For this review, take the finished solid that the model builds, in its own axes (mm). A direction names the side the tool comes from. Give positions to 0.01 mm unless a question says otherwise; leave off trailing zeros. Order: outer loops, then holes, each group sorted by start corner. A loop starts at its lowest first (then second) coordinate and runs counter-clockwise, first axis right, second up.
from build123d import *

# Parameters (mm, degrees)
SKETCH2_R               = 1.778
BOSS_EXTRUDE1_DEPTH     = 22.352
CUT_EXTRUDE1_DEPTH      = 186.610228447
CUT_EXTRUDE1_DEPTH_BACK = 186.610228447
SKETCH3_W               = 63.5
SKETCH3_H               = 9.652


with BuildPart() as part:
    # Sketch2 → Boss-Extrude1 (new body)
    with BuildSketch(Plane.XY):
        with BuildLine():
            Line((0, 6.35), (177.8, 6.35))
            ThreePointArc((177.8, 6.35), (184.15, 0), (177.8, -6.35))
            Line((177.8, -6.35), (0, -6.35))
            ThreePointArc((0, -6.35), (-6.35, 0), (0, 6.35))
        make_face()
        Circle(SKETCH2_R, mode=Mode.SUBTRACT)
        with Locations((25.4, 0)):
            Circle(SKETCH2_R, mode=Mode.SUBTRACT)
        with Locations((38.1, 0)):
            Circle(SKETCH2_R, mode=Mode.SUBTRACT)
        with Locations((50.8, 0)):
            Circle(SKETCH2_R, mode=Mode.SUBTRACT)
        with Locations(Location((127, 0, 0), (0, 0, 180))):
            Circle(SKETCH2_R, mode=Mode.SUBTRACT)
        with Locations(Location((139.7, 0, 0), (0, 0, 180))):
            Circle(SKETCH2_R, mode=Mode.SUBTRACT)
        with Locations(Location((152.4, 0, 0), (0, 0, 180))):
            Circle(SKETCH2_R, mode=Mode.SUBTRACT)
        with Locations(Location((177.8, 0, 0), (0, 0, 180))):
            Circle(SKETCH2_R, mode=Mode.SUBTRACT)
    extrude(amount=BOSS_EXTRUDE1_DEPTH)

    # Sketch3 → Cut-Extrude1 (cut, two sides: drawn at the far end of the back side and taken through both)
    with BuildSketch(Plane(origin=(0, 0, 0), x_dir=(1, 0, 0), z_dir=(0, 1, 0)).offset(-CUT_EXTRUDE1_DEPTH_BACK)):
        with Locations((25.4, -11.176)):
            Rectangle(SKETCH3_W, SKETCH3_H)
        with Locations((152.4, -11.176)):
            Rectangle(SKETCH3_W, SKETCH3_H)
    extrude(amount=CUT_EXTRUDE1_DEPTH + CUT_EXTRUDE1_DEPTH_BACK, mode=Mode.SUBTRACT)


solid = part.part
1) Clearance check with flat-ended pins moving along their axes: pin 1 (3 mm diameter, centred on y = 3, z = 13.5, fed in from +X); pin 2 (2 mm diameter, centred on x = 177.8, y = 0, fed in from +Z); pin 3 (1 mm diameter, centred on y = -0.5, z = 15, fed in from -X); pin 4 (2 mm diameter, centred on y = -4, z = 17, fed in from +X). State where each tip first meets the part, or that it passes through.
Answer sheet:
pin 1: stops at x = 120.65
pin 2: passes through
pin 3: stops at x = 57.15
pin 4: stops at x = 183.4
2) We need section B-B on x = 152.4. Give the boundary of the cut face in (y, z).
Answer sheet:
outline: (-6.35, 0) - (-1.78, 0) - (-1.78, 6.35) - (-6.35, 6.35) - close; (-6.35, 16) - (-1.78, 16) - (-1.78, 22.35) - (-6.35, 22.35) - close; (1.78, 0) - (6.35, 0) - (6.35, 6.35) - (1.78, 6.35) - close; (1.78, 16) - (6.35, 16) - (6.35, 22.35) - (1.78, 22.35) - close
3) We need section A-A on x = 11. Give the boundary of the cut face in (y, z).
Answer sheet:
outline: (-6.35, 0) - (6.35, 0) - (6.35, 6.35) - (-6.35, 6.35) - close; (-6.35, 16) - (6.35, 16) - (6.35, 22.35) - (-6.35, 22.35) - close
4) Draft analysis for pull direction X (two halves, no side actions). For faces 1 (the face through (184.15, 0.14, 19.13)), 2 (the face through (57.15, 0, 11)), 3 (the face through (154.176, -0.078, 19.133)), 4 (the face through (25, -3, 16.002)), state which applies: +X half, -X half, draft (parallel to the pull), parting line (faces both ways), or undercut.
Answer sheet:
face 1: +X half
face 2: -X half
face 3: undercut
face 4: draft
5) Tool access review of faces 5 (the face through (152, -3, 16.002)), 6 (the face through (90, 0, 0)): name each direction out of +Z, -Z, +X, -X, +Y, -Y from which nothing blocks a thin tool from reaching the whole face with its end or side.
Answer sheet:
face 5: +X, +Y, -Y
face 6: -Z, +X, -X, +Y, -Y
6) We need section C-C on y = 0. Count the separate pieces of the cut face and the enclosed holes in it, then the cut area to 3 significant figures.
Answer sheet:
separate pieces: 17
enclosed holes: 0
area: 2,670 mm2
7) To check wall thickness, follow line 1 (Z direction, x = 166.5, y = 1.25); line 2 (Y direction, x = 152.4, z = 4.25). State the ranges of each line that lie inside material, in increasing order.
Answer sheet:
line 1: z = 0 to 6.35, 16 to 22.35
line 2: y = -6.35 to -1.78, 1.78 to 6.35
8) We need section D-D on z = 9.5. Give the boundary of the cut face in (x, y), then the cut area to 3 significant figures.
Answer sheet:
outline: (57.15, -6.35) - (120.65, -6.35) - (120.65, 6.35) - (57.15, 6.35) - close
area: 806 mm2
